For this review, use the dimensioned drawing (mm, ordinates from the lowest corner) and the shaded views. Coordinates: 2 decimals unless noted, no trailing zeros. Write each loop counter-clockwise with the first axis right and the second up, starting at its lowest first coordinate (ties: lowest second). Pieces come first, ordered by that corner, then holes. Notation, with made-up numbers: (-8.5, -18) - (0.5, -18) arc R30 cw to (0.5, 10) - close; hole circle Ø6 at (55, 8). An arc over 180 degrees is marked (long way). One line per item, written item: value.
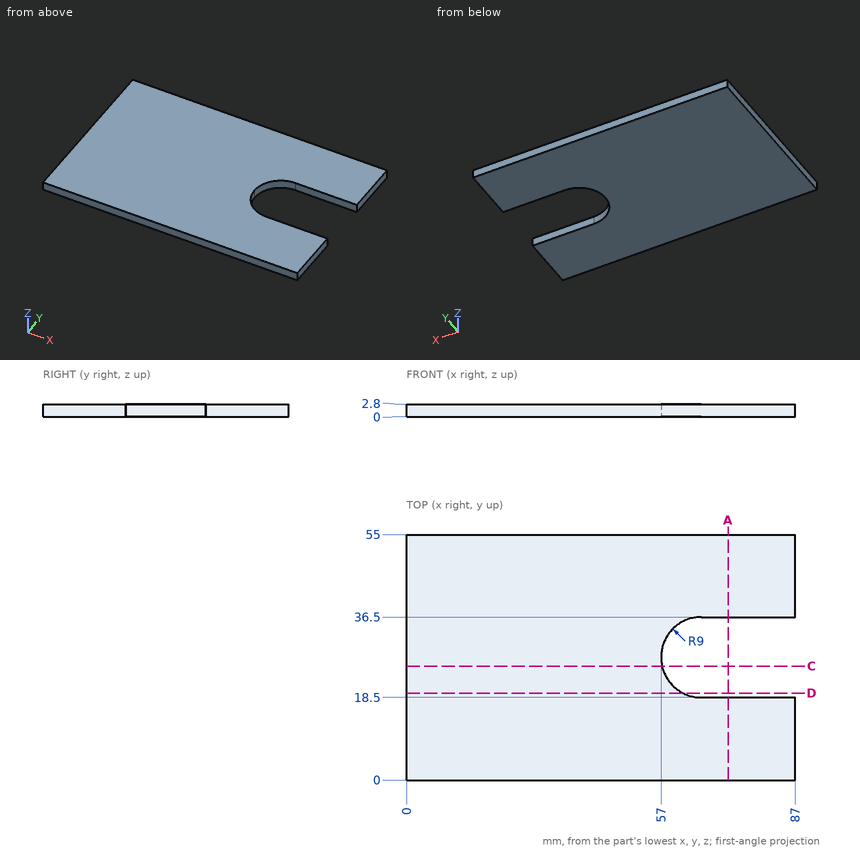
1. Consider section A-A, the plane x = 72. Write out the cut boundary in (y, z).
Answer block:
outline: (0, 0) - (18.5, 0) - (18.5, 2.8) - (0, 2.8) - close; (36.5, 0) - (55, 0) - (55, 2.8) - (36.5, 2.8) - close
2. Consider section C-C, the plane y = 25.5. Write out the cut boundary in (x, z), then the cut area to 3 significant figures.
Answer block:
outline: (0, 0) - (57.23, 0) - (57.23, 2.8) - (0, 2.8) - close
area: 160 mm^2
3. Consider section D-D, the plane y = 19.5. Write out the cut boundary in (x, z).
Answer block:
outline: (0, 0) - (61.88, 0) - (61.88, 2.8) - (0, 2.8) - close
4. Wall thickness on line 1 along Y through (x, z) = (68.5, 1.1); line 2 along Y through (x, z) = (60, 0.7); line 3 along X through (y, z) = (34.5, 0.65): over which ranges is each line inside the solid? List them lowest first.
Answer block:
line 1: y = 0 to 18.5, 36.5 to 55
line 2: y = 0 to 20.79, 34.21 to 55
line 3: x = 0 to 60.34
